Input: part model. Units: mm. Frame: model coordinates. Face numbers are marked on the shaded views. A direction names the side the tool comes from. Round coordinates to 2 decimals unless told otherwise and drop trailing zeros. Loops run counter-clockwise (first coordinate to the right, second up) from the corner with the lowest first, then second, coordinate; pieces in that order, holes last. Notation, with made-up numbers: (51.5, -1.75) - (100.5, -1.75) arc R15 cw to (100.5, 27.25) - close; hole circle Ø8 at (84, 29.25). An arc over 180 degrees is marked (long way). One line per question, with ' | ' between items. Start each with the question number.
Item 1: First-contact query: pin 1 (2 mm diameter, centred on x = -2.5, z = 0, fed in from +Y); pin 2 (4.5 mm diameter, centred on y = -14.5, z = -3, fed in from -X); pin 3 (7.5 mm diameter, centred on x = 5.5, z = -1, fed in from +Y). Flat tips, straight axial feed; report the tip coordinate or a pass-through.
Item 2: Set-up query: the marked faces 1, 2 and 3. Return all of +Z, -Z, +X, -X, +Y, -Y with unobstructed straight access to the full face (end or side cutting, diameter ignored); none if empty.
Item 3: Section A-A, the plane y = 0. Return loops of the section in (x, z) (3 decimals), plus the area to 3 significant figures.
Item 4: Section C-C, the plane z = -7.75. Return loops of the section in (x, y).
Item 5: Draft query along Y for the marked faces 4, 5 and 6. Return one class per face: pulls with the +Y half, pulls with the -Y half, needs draft (parallel to the pull), parting line crosses it, or undercut.
Item 6: Material intervals for line 1 along Y through (x, z) = (-35, 4.25); line 2 along X through (y, z) = (6.5, 4.75); line 3 along Y through (x, z) = (0, 5.75), sorted ascending.
Item 7: Section D-D, the plane y = -8. Return loops of the section in (x, z) (3 decimals), plus the area to 3 significant figures.
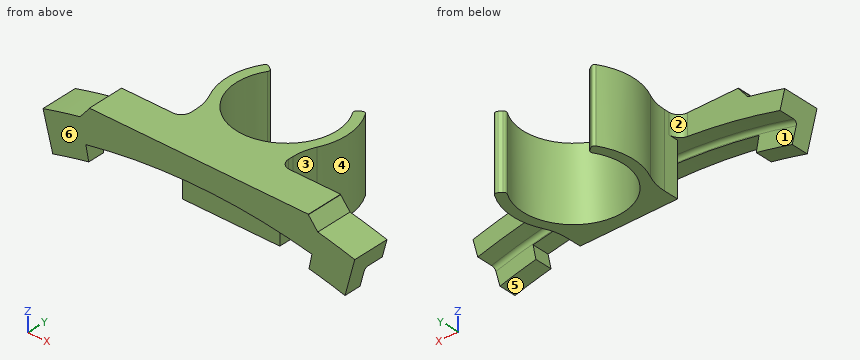
```python
from build123d import *

# Parameters (mm, degrees)
F1_DEPTH       = 9.525
F2_DEPTH       = 9.525
F3_T1_DEPTH    = 19.05
F3_T3_DEPTH    = 9.525
F3_T5_DEPTH    = 9.525
F4_R           = 0.762
F6_W           = 9.525
F6_H           = 3.81
F6_W_2         = 4.445
F7_ANGLE_BACK  = 15
F7_ANGLE       = 30
F8_R           = 1.016
F9_DEPTH       = 28.575
F10_R          = 2.54
F11_T1_DEPTH   = 9.525
F12_ANGLE_BACK = 11.25
F12_ANGLE      = 22.5


# Not quite as in the source:
# - a fillet or chamfer that OpenCascade refuses, or shapes differently, is made with other operations: its cross-section is extruded or revolved along the edge and cut away or added


with BuildPart() as f1:
    # F0 (on Top) → F1 (new body, symmetric)
    with BuildSketch(Plane.XY):
        with BuildLine():
            ThreePointArc((12.7, -9.0953637091), (14.8728333044, -4.7764495705), (15.621, 0))
            ThreePointArc((15.621, 0), (14.8980124876, 4.6973252941), (12.7959740838, 8.9598375122))
            Line((12.7959740838, 8.9598375122), (10.7153278913, 7.5029533639))
            ThreePointArc((10.7153278913, 7.5029533639), (12.4755714327, 3.9335325633), (13.081, 0))
            ThreePointArc((13.081, 0), (-3.9335325633, -12.4755714327), (-10.7153278913, 7.5029533639))
            Line((-10.7153278913, 7.5029533639), (-12.7959740838, 8.9598375122))
            ThreePointArc((-12.7959740838, 8.9598375122), (-15.6207793149, -0.0830336901), (-12.7, -9.0953637091))
            ThreePointArc((-12.7, -9.0953637091), (0, -15.621), (12.7, -9.0953637091))
        make_face()
    extrude(amount=F1_DEPTH, both=True)

    # F0 (on Top) → F2 (join, symmetric)
    with BuildSketch(Plane.XY):
        with BuildLine():
            Line((12.7, -16.4338), (12.7, -9.0953637091))
            ThreePointArc((12.7, -9.0953637091), (0, -15.621), (-12.7, -9.0953637091))
            Line((-12.7, -9.0953637091), (-12.7, -16.4338))
            Line((-12.7, -16.4338), (12.7, -16.4338))
        make_face()
    extrude(amount=F2_DEPTH, both=True)

    # F3: fillet of radius 12.7 on 3 edges, made by hand

    # F3_s2 → F3_t1 (join)
    with BuildSketch(Plane.XY.offset(-9.525)):
        with BuildLine():
            ThreePointArc((-14.0098654709, -6.9093639714), (-13.0318006864, -9.6427001587), (-12.7, -12.5267330538))
            Line((-12.7, -12.5267330538), (-12.7, -9.0953637091))
            ThreePointArc((-12.7, -9.0953637091), (-13.3995849593, -8.0291197475), (-14.0098654709, -6.9093639714))
        make_face()
    extrude(amount=F3_T1_DEPTH)

    # F3_s4 → F3_t3 (join)
    with BuildSketch(Plane.XY):
        with BuildLine():
            ThreePointArc((14.0098654709, -6.9093639714), (13.0318006864, -9.6427001587), (12.7, -12.5267330538))
            Line((12.7, -12.5267330538), (12.7, -9.0953637091))
            ThreePointArc((12.7, -9.0953637091), (13.3995849593, -8.0291197475), (14.0098654709, -6.9093639714))
        make_face()
    extrude(amount=F3_T3_DEPTH)

    # F3_s6 → F3_t5 (join)
    with BuildSketch(Plane.XY.offset(-9.525)):
        with BuildLine():
            ThreePointArc((12.7, -12.5267330538), (13.0318006864, -9.6427001587), (14.0098654709, -6.9093639714))
            ThreePointArc((14.0098654709, -6.9093639714), (13.3995849593, -8.0291197475), (12.7, -9.0953637091))
            Line((12.7, -9.0953637091), (12.7, -12.5267330538))
        make_face()
    extrude(amount=F3_T5_DEPTH)

    # F4
    f4_edges = [f1.edges().sort_by_distance(p)[0] for p in [
        (-12.795974, 8.959838, 0),
        (-10.715328, 7.502953, -4.7625),
        (-10.715328, 7.502953, 4.7625),
        (12.795974, 8.959838, 4.7625),
        (12.795974, 8.959838, -4.7625),
        (10.715328, 7.502953, 4.7625),
        (10.715328, 7.502953, -4.7625),
    ]]
    fillet(f4_edges, radius=F4_R)

    # F6 (on Right) → F7 (revolve)
    with BuildSketch(Plane.YZ, mode=Mode.PRIVATE) as f7_sk:
        with Locations((-21.1963, 7.62)):
            Rectangle(F6_W, F6_H)
        Polygon((-16.4338, 4.7625), (-16.4338, 5.715), (-25.9588, 5.715), (-25.9588, 3.4925), (-21.5138, 3.4925), (-21.5138, 4.7625), align=None)
        with Locations((-23.7363, 1.5875)):
            Rectangle(F6_W_2, F6_H)
    revolve(f7_sk.sketch.rotate(Axis((0, -16.4338, -147.6375), (0, -1, 0)), -F7_ANGLE_BACK), axis=Axis((0, -16.4338, -147.6375), (0, -1, 0)), revolution_arc=F7_ANGLE)

    # F8
    f8_edges = [f1.edges().sort_by_distance(p)[0] for p in [
        (0, -21.5138, 4.7625),
    ]]
    fillet(f8_edges, radius=F8_R)

    # F6 (on Right) → F9 (join, symmetric)
    with BuildSketch(Plane.YZ):
        with Locations((-21.1963, 7.62)):
            Rectangle(F6_W, F6_H)
        Polygon((-16.4338, 4.7625), (-16.4338, 5.715), (-25.9588, 5.715), (-25.9588, 3.4925), (-21.5138, 3.4925), (-21.5138, 4.7625), align=None)
        with Locations((-23.7363, 1.5875)):
            Rectangle(F6_W_2, F6_H)
    extrude(amount=F9_DEPTH, both=True)

    # F10
    f10_edges = [f1.edges().sort_by_distance(p)[0] for p in [
        (-12.7, -16.4338, 6.878706),
        (12.7, -16.4338, 6.878706),
    ]]
    fillet(f10_edges, radius=F10_R)

    # F11: chamfer of 2.54 on 2 edges, made by hand

    # F11_s2 → F11_t1 (join)
    with BuildSketch(Plane.XZ.offset(16.4338)):
        with BuildLine():
            Line((-31.089435357, 6.3536630782), (-28.5106384895, 9.503518522))
            Line((-28.5106384895, 9.503518522), (-28.4598384895, 9.503518522))
            ThreePointArc((-28.4598384895, 9.503518522), (-28.5242, 8.2044800333), (-28.5242, 6.9054415446))
            Line((-28.5242, 6.9054415446), (-28.5657636364, 6.8554882705))
            ThreePointArc((-28.5657636364, 6.8554882705), (-29.8296810134, 6.6164348202), (-31.0794070503, 6.3038627463))
            Line((-31.0794070503, 6.3038627463), (-31.089435357, 6.3536630782))
        make_face()
        with BuildLine():
            Line((31.089435357, 6.3536630782), (28.5106384895, 9.503518522))
            Line((28.5106384895, 9.503518522), (28.4598384895, 9.503518522))
            ThreePointArc((28.4598384895, 9.503518522), (28.5242, 8.2044800333), (28.5242, 6.9054415446))
            Line((28.5242, 6.9054415446), (28.5657636364, 6.8554882705))
            ThreePointArc((28.5657636364, 6.8554882705), (29.8296810134, 6.6164348202), (31.0794070503, 6.3038627463))
            Line((31.0794070503, 6.3038627463), (31.089435357, 6.3536630782))
        make_face()
    extrude(amount=F11_T1_DEPTH)

    # F6 (on Right) → F12 (revolve, cut)
    with BuildSketch(Plane.YZ, mode=Mode.PRIVATE) as f12_sk:
        with Locations((-23.7363, 1.5875)):
            Rectangle(F6_W_2, F6_H)
    revolve(f12_sk.sketch.rotate(Axis((0, -25.9588, -147.6375), (0, 1, 0)), -F12_ANGLE_BACK), axis=Axis((0, -25.9588, -147.6375), (0, 1, 0)), revolution_arc=F12_ANGLE, mode=Mode.SUBTRACT)


solid = f1.part
```
Return value:
1) pin 1: y = -12.6 | pin 2: x = -12.7 | pin 3: y = -9.25
2) face 1: -Z | face 2: +Z, -Z, -X | face 3: +Z, -Z, +X
3) outline: (-15.621, -9.525) - (-13.081, -9.525) - (-13.081, 9.525) - (-15.621, 9.525) - close; (13.081, -9.525) - (15.621, -9.525) - (15.621, 9.525) - (13.081, 9.525) - close | area: 96.8 mm2
4) outline: (-14.01, -6.91) arc R12.7 cw to (-12.7, -12.53) - (-12.7, -16.43) - (12.7, -16.43) - (12.7, -12.53) arc R12.7 cw to (14.01, -6.91) arc R15.62 ccw to (13.24, 8.29) arc R0.76 ccw to (12.16, 8.51) - (11.32, 7.93) arc R0.76 ccw to (11.11, 6.9) arc R13.08 cw (long way) to (-11.11, 6.9) arc R0.76 ccw to (-11.32, 7.93) - (-12.16, 8.51) arc R0.76 ccw to (-13.24, 8.29) arc R15.62 ccw to start
5) face 4: undercut | face 5: needs draft | face 6: pulls with the -Y half
6) line 1: -25.96 to -16.43 | line 2: -14.2 to -11.35, 11.35 to 14.2 | line 3: -25.96 to -13.08
7) outline: (-13.534, -9.525) - (-10.35, -9.525) - (-10.35, 9.525) - (-13.534, 9.525) - close; (10.35, -9.525) - (13.534, -9.525) - (13.534, 9.525) - (10.35, 9.525) - close | area: 121 mm2
